```python
from build123d import *

# Parameters (mm, degrees)
SKICA1_R                 = 1.5
P_IDAT_VYSUNUT_M1_DEPTH  = 4
SKICA2_W                 = 7.826237638
SKICA2_H                 = 4
P_IDAT_VYSUNUT_M2_DEPTH  = 16
SKICA3_W                 = 7.826237638
SKICA3_H                 = 24
SKICA3_R                 = 2.5
P_IDAT_VYSUNUT_M3_DEPTH  = 4
SKICA4_W                 = 5.18826407
SKICA4_H                 = 5
ODEBRAT_VYSUNUT_M1_DEPTH = 4
ZAOBLIT1_R               = 1
ZAOBLIT2_R               = 1


with BuildPart() as part:
    # Skica1 → Přidat vysunutím1 (new body)
    with BuildSketch(Plane.XY):
        with BuildLine():
            Line((108.413118819, 104.5), (108.413118819, 82.5))
            Line((108.413118819, 82.5), (100.586881181, 82.5))
            Line((100.586881181, 82.5), (100.586881181, 104.5))
            ThreePointArc((100.586881181, 104.5), (104.5, 108.413118819), (108.413118819, 104.5))
        make_face()
        with Locations((104.5, 104.5)):
            Circle(SKICA1_R, mode=Mode.SUBTRACT)
    extrude(amount=P_IDAT_VYSUNUT_M1_DEPTH)

    # Skica2 → Přidat vysunutím2 (add)
    with BuildSketch(Plane.XY.offset(4)):
        with Locations((104.5, 84.5)):
            Rectangle(SKICA2_W, SKICA2_H)
    extrude(amount=P_IDAT_VYSUNUT_M2_DEPTH)

    # Skica3 → Přidat vysunutím3 (add)
    with BuildSketch(Plane.XY.offset(20)):
        with Locations((104.5, 74.5)):
            Rectangle(SKICA3_W, SKICA3_H)
        with Locations((104.5, 72.5)):
            Circle(SKICA3_R, mode=Mode.SUBTRACT)
    extrude(amount=P_IDAT_VYSUNUT_M3_DEPTH)

    # Skica4 → Odebrat vysunutím1 (cut)
    with BuildSketch(Plane(origin=(0, 86.5, 0), x_dir=(1, 0, 0), z_dir=(0, 1, 0))):
        with Locations((105.818986784, -9.982223616)):
            Rectangle(SKICA4_W, SKICA4_H)
    extrude(amount=-ODEBRAT_VYSUNUT_M1_DEPTH, mode=Mode.SUBTRACT)

    # Zaoblit1
    zaoblit1_edges = [part.edges().sort_by_distance(p)[0] for p in [
        (104.5, 86.5, 24),
    ]]
    fillet(zaoblit1_edges, radius=ZAOBLIT1_R)

    # Zaoblit2
    zaoblit2_edges = [part.edges().sort_by_distance(p)[0] for p in [
        (104.5, 62.5, 24),
        (104.5, 62.5, 20),
        (100.586881181, 62.5, 22),
        (108.413118819, 62.5, 22),
        (104.5, 82.5, 0),
    ]]
    fillet(zaoblit2_edges, radius=ZAOBLIT2_R)


solid = part.part
```
For this review, take the finished solid that the model builds, in its own axes (mm). A direction names the side the tool comes from. Coordinates: 2 decimals unless noted, no trailing zeros. Order: outer loops, then holes, each group sorted by start corner. A loop starts at its lowest first (then second) coordinate and runs counter-clockwise, first axis right, second up. Notation, with made-up numbers: (-32.75, -28.75) -> (18.25, -28.75) arc R13 cw to (18.25, -24.75) -> close; hole circle Ø5 at (4, 71). An arc over 180 degrees is marked (long way). Use CSV: the item, a comma, the result in double quotes. Start each with the question number.
Item 1: Draft analysis for pull direction Y (two halves, no side actions). For faces 4 (the face through (104.4, 75.2, 20)), 5 (the face through (104, 86.5, 13)), 6 (the face through (105.65, 70.28, 21.97)), state which applies: pulls with the +Y half, pulls with the -Y half, needs draft (parallel to the pull), parting line crosses it, or undercut.
Item 2: Wall thickness on probe 1 along X at (y, z) = (104.5, 2.1); probe 2 along Y at (x, z) = (104.5, 22.2); probe 3 along Y at (x, z) = (104.5, 1.2): over which ranges is each line inside the solid? List them lowest first.
Item 3: We need section A-A, the plane x = 104.5. Give the boundary of the cut face in (y, z), then the cut area to 3 significant figures.
Item 4: We need section D-D, the plane x = 106.5. Give the boundary of the cut face in (y, z), then the cut area to 3 significant figures.
Item 5: We need section C-C, the plane z = 2.75. Give the boundary of the cut face in (x, y).
Item 6: We need section B-B, the plane y = 72.5. Give the boundary of the cut face in (x, z), then the cut area to 3 significant figures.
Item 7: For faces 1 (the face through (108.413, 77, 21)), 2 (the face through (106, 85, 12.482)), 3 (the face through (105, 98, 4)), list the 3-axis set-ups (+Z, -Z, +X, -X, +Y, -Y) from which the entire face can be reached by the end or side of a thin tool; tool diameter is ignored.
Item 8: Insertion check: pin 1 (2 mm diameter, centred on x = 105.5, y = 88, fed in from +Z); pin 2 (3 mm diameter, centred on y = 84.5, z = 10, fed in from +X); pin 3 (2 mm diameter, centred on x = 107, z = 18, fed in from +Y). Each pin has a flat end and moves straight along its axis. Give the tip position at first contact, or say it passes through.
Derived:
1,face 4,"needs draft"
1,face 5,"pulls with the +Y half"
1,face 6,"undercut"
2,probe 1,"x = 100.59 to 103, 106 to 108.41"
2,probe 2,"y = 62.5 to 70, 75 to 86.5"
2,probe 3,"y = 82.5 to 103, 106 to 108.41"
3,outline,"(62.5, 21) arc R1 ccw to (63.5, 20) -> (70, 20) -> (70, 24) -> (63.5, 24) arc R1 ccw to (62.5, 23) -> close; (75, 20) -> (82.5, 20) -> (82.5, 12.48) -> (86.5, 12.48) -> (86.5, 23) arc R1 ccw to (85.5, 24) -> (75, 24) -> close; (82.5, 1) arc R1 ccw to (83.5, 0) -> (103, 0) -> (103, 4) -> (86.5, 4) -> (86.5, 7.48) -> (82.5, 7.48) -> close; (106, 0) -> (108.41, 0) -> (108.41, 4) -> (106, 4) -> close"
3,area,"211 mm^2"
4,outline,"(62.5, 21) arc R1 ccw to (63.5, 20) -> (71, 20) -> (71, 24) -> (63.5, 24) arc R1 ccw to (62.5, 23) -> close; (74, 20) -> (82.5, 20) -> (82.5, 12.48) -> (86.5, 12.48) -> (86.5, 23) arc R1 ccw to (85.5, 24) -> (74, 24) -> close; (82.5, 1) arc R1 ccw to (83.5, 0) -> (107.86, 0) -> (107.86, 4) -> (86.5, 4) -> (86.5, 7.48) -> (82.5, 7.48) -> close"
4,area,"229 mm^2"
5,outline,"(100.59, 82.5) -> (108.41, 82.5) -> (108.41, 104.5) arc R3.91 ccw to (100.59, 104.5) -> close; hole circle Ø3 at (104.5, 104.5)"
6,outline,"(100.59, 20) -> (102, 20) -> (102, 24) -> (100.59, 24) -> close; (107, 20) -> (108.41, 20) -> (108.41, 24) -> (107, 24) -> close"
6,area,"11.3 mm^2"
7,face 1,"+Z, -Z, +X, +Y, -Y"
7,face 2,"+X, +Y, -Y"
7,face 3,"+Z, +X, -X, +Y"
8,pin 1,"stops at z = 4"
8,pin 2,"stops at x = 103.22"
8,pin 3,"stops at y = 86.5"
